```python
from build123d import *

# Parameters (mm, degrees)
SKETCH_1_R          = 4
EXTRUDE_1_DEPTH     = 12
SKETCH_2_R          = 2.7
CUT_EXTRUDE_1_DEPTH = 4.2
SKETCH_3_OUTSIDE_W  = 13.298
SKETCH_3_OUTSIDE_H  = 13.298
SKETCH_3_OUTSIDE_R  = 3.2
CUT_EXTRUDE_2_DEPTH = 11.2
SKETCH_4_R          = 1.6
CUT_EXTRUDE_3_DEPTH = 11.2
CHAMFER_1_SIZE      = 0.2


with BuildPart() as part:
    # Эскиз1 → Бобышка-Вытянуть1 (new body)
    with BuildSketch(Plane.XY):
        Circle(SKETCH_1_R)
    extrude(amount=EXTRUDE_1_DEPTH)

    # Эскиз2 → Вырез-Вытянуть1 (cut)
    with BuildSketch(Plane.XY.offset(12)):
        Circle(SKETCH_2_R)
    extrude(amount=-CUT_EXTRUDE_1_DEPTH, mode=Mode.SUBTRACT)

    # Эскиз3 outside → Вырез-Вытянуть2 (cut)
    with BuildSketch(Plane(origin=(0, 0, 0), x_dir=(-1, 0, 0), z_dir=(0, 0, -1))):
        Rectangle(SKETCH_3_OUTSIDE_W, SKETCH_3_OUTSIDE_H)
        Circle(SKETCH_3_OUTSIDE_R, mode=Mode.SUBTRACT)
    extrude(amount=-CUT_EXTRUDE_2_DEPTH, mode=Mode.SUBTRACT)

    # Эскиз4 → Вырез-Вытянуть3 (cut)
    with BuildSketch(Plane(origin=(0, 0, 0), x_dir=(-1, 0, 0), z_dir=(0, 0, -1))):
        Circle(SKETCH_4_R)
    extrude(amount=-CUT_EXTRUDE_3_DEPTH, mode=Mode.SUBTRACT)

    # Фаска1
    chamfer_1_edges = [part.edges().sort_by_distance(p)[0] for p in [
        (3.2, 0, 0),
    ]]
    chamfer(chamfer_1_edges, length=CHAMFER_1_SIZE)


solid = part.part
```
Here's how the part is built. I have some questions about the finished solid (model axes, mm). A direction names the side the tool comes from. Coordinates: 2 decimals unless noted, no trailing zeros. Order: outer loops, then holes, each group sorted by start corner. A loop starts at its lowest first (then second) coordinate and runs counter-clockwise, first axis right, second up.
1) We'd pull the mould along Y, two halves only. Please class faces 1 (the face through (2, 3, 11.2)), 2 (the face through (1.27, -0.97, 3.85)), 3 (the face through (-0.867, -3.905, 11.594)): +Y half, -Y half, draft (parallel to the pull), parting line (faces both ways), or undercut.
2) Imagine slicing it at D-D on y = 3.5. List the corners of the cut face in (x, z) for me.
3) Imagine slicing it at C-C on z = 8. List the corners of the cut face in (x, y) for me.
4) Which directions (+Z, -Z, +X, -X, +Y, -Y) give clear straight access to the entire face, cutting with the end or side of a thin tool? Please do faces 4 (the face through (2.539, -1.947, 5.623)), 5 (the face through (3, -1, 12)), 6 (the face through (0, -2, 7.8)).
5) Imagine slicing it at A-A on y = 0. List the corners of the cut face in (x, z) for me, and give its area (3 significant figures).
6) I need wall thicknesses on line 1 (Y direction, x = 0, z = 8.75); line 2 (Z direction, x = 0.5, y = 2.5); line 3 (Z direction, x = -1.5, y = -3). Which ranges of each line are inside material? Lowest first, please.
7) Will these pins go through, and if not, where does the flat tip stop? pin 1 (3 mm diameter, centred on x = 1, z = 1.5, fed in from -Y); pin 2 (2.5 mm diameter, centred on x = 0, y = 0, fed in from +Z); pin 3 (4 mm diameter, centred on y = -2, z = 6, fed in from -X); pin 4 (4.5 mm diameter, centred on x = 0, y = 0, fed in from +Z).
Response values:
1. face 1: draft
1. face 2: undercut
1. face 3: parting line
2. outline: (-1.94, 11.2) - (1.94, 11.2) - (1.94, 12) - (-1.94, 12) - close
3. outline: circle Ø6.4 at (0, 0); hole circle Ø5.4 at (0, 0)
4. face 4: -Z
4. face 5: +Z, +X, -X, +Y, -Y
4. face 6: +Z
5. outline: (-4, 11.2) - (-3.2, 11.2) - (-3.2, 0.2) - (-3, 0) - (-1.6, 0) - (-1.6, 7.8) - (-2.7, 7.8) - (-2.7, 12) - (-4, 12) - close; (1.6, 0) - (3, 0) - (3.2, 0.2) - (3.2, 11.2) - (4, 11.2) - (4, 12) - (2.7, 12) - (2.7, 7.8) - (1.6, 7.8) - close
5. area: 30.4 mm2
6. line 1: y = -3.2 to -2.7, 2.7 to 3.2
6. line 2: z = 0 to 7.8
6. line 3: z = 11.2 to 12
7. pin 1: stops at y = -3.2
7. pin 2: passes through
7. pin 3: stops at x = -3.2
7. pin 4: stops at z = 7.8
